from build123d import *

# Parameters (mm, degrees)
F0_R     = 9.5
F1_DEPTH = 3
F2_R     = 4.05
F3_DEPTH = 4.5
F4_SIZE  = 0.5
F5_R     = 4.55
F6_DEPTH = 1.5


with BuildPart() as f1:
    # F0 (on Top) → F1 (new body)
    with BuildSketch(Plane.XY):
        Circle(F0_R)
    extrude(amount=F1_DEPTH)

    # F2 (on face) → F3 (join)
    with BuildSketch(Plane.XY.offset(3)):
        Circle(F2_R)
    extrude(amount=F3_DEPTH)

    # F4
    f4_edges = [f1.edges().sort_by_distance(p)[0] for p in [
        (-4.05, 0, 7.5),
        (-9.5, 0, 3),
        (-9.5, 0, 0),
    ]]
    chamfer(f4_edges, length=F4_SIZE)

    # F5 (on face) → F6 (join)
    with BuildSketch(Plane.XY.offset(3)):
        Circle(F5_R)
    extrude(amount=F6_DEPTH)


solid = f1.part
The model under review builds one solid part; all positions refer to its coordinate system, in mm. A direction names the side the tool comes from. Give positions to 0.01 mm unless a question says otherwise; leave off trailing zeros. Loops run counter-clockwise (first coordinate to the right, second up) from the corner with the lowest first, then second, coordinate; pieces in that order, holes last. Notation, with made-up numbers: (49.5, 57.5) -> (59.5, 57.5) arc R31 ccw to (59.5, 89.5) -> close; hole circle Ø4 at (67.25, 54). An arc over 180 degrees is marked (long way). Answer as a JSON object with one key per item and string values. Group by question number.
Q1. Insertion check: pin 1 (1.5 mm diameter, centred on y = 2.5, z = 4, fed in from +X). The pin has a flat end and moves straight along its axis. Give the tip position at first contact, or say it passes through.
Q2. Tool access review of faces 1 (the cylindrical face through (4.38, -8.43, 1.49)), 2 (the cylindrical face through (-0.878, -3.954, 5.732)): name each direction out of +Z, -Z, +X, -X, +Y, -Y from which nothing blocks a thin tool from reaching the whole face with its end or side.
Q3. Take a section at D-D (z = 3.5). Write out the cut boundary in (x, y).
Q4. Take a section at A-A (y = 0). Write out the cut boundary in (x, z).
Q5. Take a section at C-C (z = 6.25). Write out the cut boundary in (x, y).
Q6. Wall thickness on line 1 along Z through (x, y) = (-3.5, -4.25); line 2 along Y through (x, z) = (-0.25, 1.5); line 3 along X through (y, z) = (1, 2): over which ranges is each line inside the solid? List them lowest first.
Answer below:
{
 "1": {"pin 1": "stops at x = 4.2"},
 "2": {"face 1": "+Z, -Z", "face 2": "+Z"},
 "3": {"outline": "circle Ø9.1 at (0, 0)"},
 "4": {"outline": "(-9.5, 0.5) -> (-9, 0) -> (9, 0) -> (9.5, 0.5) -> (9.5, 2.5) -> (9, 3) -> (4.55, 3) -> (4.55, 4.5) -> (4.05, 4.5) -> (4.05, 7) -> (3.55, 7.5) -> (-3.55, 7.5) -> (-4.05, 7) -> (-4.05, 4.5) -> (-4.55, 4.5) -> (-4.55, 3) -> (-9, 3) -> (-9.5, 2.5) -> close"},
 "5": {"outline": "circle Ø8.1 at (0, 0)"},
 "6": {"line 1": "z = 0 to 3", "line 2": "y = -9.5 to 9.5", "line 3": "x = -9.45 to 9.45"}
}
